```python
from build123d import *

# Parameters (mm, degrees)
BOX018_W     = 31
BOX018_H     = 68
BOX018_DEPTH = 12
FILLET010_R  = 15
FILLET011_R  = 2


with BuildPart() as part:
    # Box018 → Box018 (new body)
    with BuildSketch(Plane(origin=(-15.5, -34, 1.7), x_dir=(1, 0, 0), z_dir=(0, 0, 1))):
        with Locations((15.5, 34)):
            Rectangle(BOX018_W, BOX018_H)
    extrude(amount=BOX018_DEPTH)

    # Fillet010
    fillet010_edges = [part.edges().sort_by_distance(p)[0] for p in [
        (-15.5, -34, 7.7),
        (-15.5, 34, 7.7),
        (15.5, -34, 7.7),
        (15.5, 34, 7.7),
    ]]
    fillet(fillet010_edges, radius=FILLET010_R)

    # Fillet011
    fillet011_edges = [part.edges().sort_by_distance(p)[0] for p in [
        (-15.5, 0, 13.7),
        (-11.106602, -29.606602, 13.7),
        (-11.106602, 29.606602, 13.7),
        (0, -34, 13.7),
        (0, 34, 13.7),
        (11.106602, -29.606602, 13.7),
        (11.106602, 29.606602, 13.7),
        (15.5, 0, 13.7),
    ]]
    fillet(fillet011_edges, radius=FILLET011_R)


with BuildPart() as part_1:
    # Fillet011 placement: moved
    add(part.part.moved(Location((0, 0, 40))))


solid = part_1.part
```
The model under review builds one solid part; all positions refer to its coordinate system, in mm. Give positions to 0.01 mm unless a question says otherwise; leave off trailing zeros. Write each loop counter-clockwise with the first axis right and the second up, starting at its lowest first coordinate (ties: lowest second). Pieces come first, ordered by that corner, then holes. Notation, with made-up numbers: M 86,0 L 113,0 A17 cw 113,7 Z; hole C -32.5,-1 d7. An arc over 180 degrees is marked long. Answer in a Markdown table with one row per item.
Item 1: Add section B-B on z = 52.5. Give the boundary of the cut face in (x, y).
Check sheet entries:
| item | result |
|---|---|
| outline | M -15.33,-19 A14.83 ccw -0.5,-33.83 L 0.5,-33.83 A14.83 ccw 15.33,-19 L 15.33,19 A14.83 ccw 0.5,33.83 L -0.5,33.83 A14.83 ccw -15.33,19 Z |
Item 2: For P1, Ø3, axis at x = -10, z = 51, coming from the -Y side; P2, Ø5, axis at y = 25.5, z = 47, coming from the -X side; P3, Ø3, axis at x = -8, z = 47.5, coming from the -Y side, all flat-tipped, find the tip position at first contact; note any pin that passes through.
Check sheet entries:
| item | result |
|---|---|
| P1 | y = -31.69 |
| P2 | x = -14.96 |
| P3 | y = -32.75 |
Item 3: For line 1 along Y through (x, z) = (5, 47); line 2 along X through (y, z) = (-19.5, 51); line 3 along Y through (x, z) = (-6.5, 45.5), list the stretches that pass through material, from the lowest coordinate up.
Check sheet entries:
| item | result |
|---|---|
| line 1 | -33.31 to 33.31 |
| line 2 | -15.49 to 15.49 |
| line 3 | -32.75 to 32.75 |
Item 4: Add section A-A on z = 45.5. Give the boundary of the cut face in (x, y), plus the area to 3 significant figures.
Check sheet entries:
| item | result |
|---|---|
| outline | M -15.5,-19 A15 ccw -0.5,-34 L 0.5,-34 A15 ccw 15.5,-19 L 15.5,19 A15 ccw 0.5,34 L -0.5,34 A15 ccw -15.5,19 Z |
| area | 1,910 mm2 |
